from build123d import *

# Parameters (mm, degrees)
SKETCH_1_W          = 147
SKETCH_1_H          = 20
EXTRUDE_1_DEPTH     = 2
CUT_EXTRUDE_1_DEPTH = 3
SKETCH_3_R          = 1
CUT_EXTRUDE_2_DEPTH = 3
SKETCH_4_R          = 1.75
CUT_EXTRUDE_3_DEPTH = 3
CUT_EXTRUDE_4_DEPTH = 3


with BuildPart() as part:
    # 草图1 → 凸台-拉伸1 (new body)
    with BuildSketch(Plane.XY):
        Rectangle(SKETCH_1_W, SKETCH_1_H)
    extrude(amount=EXTRUDE_1_DEPTH)

    # 草图2 → 切除-拉伸1 (cut)
    with BuildSketch(Plane.XY.offset(2)):
        Polygon((30.510902349, 3.396971992), (30.740864968, 1.209023822), (45.658693398, 2.776950771), (45.428730779, 4.964898941), align=None)
    cut_extrude_1 = extrude(amount=-CUT_EXTRUDE_1_DEPTH, mode=Mode.SUBTRACT)

    # 草图3 → 切除-拉伸2 (cut, through all)
    with BuildSketch(Plane.XY.offset(2)):
        with Locations((31.505424244, 3.501500455)):
            Circle(SKETCH_3_R)
        with Locations((31.735386863, 1.313552286)):
            Circle(SKETCH_3_R)
        with Locations((44.434208884, 4.860370478)):
            Circle(SKETCH_3_R)
        with Locations((44.664171503, 2.672422308)):
            Circle(SKETCH_3_R)
    cut_extrude_2 = extrude(amount=-CUT_EXTRUDE_2_DEPTH, mode=Mode.SUBTRACT)

    # 镜向1: 切除-拉伸1, 切除-拉伸2 across plane
    add(cut_extrude_1.mirror(Plane(origin=(0, 0, 0), x_dir=(0, 0, 1), z_dir=(1, 0, 0))), mode=Mode.SUBTRACT)
    add(cut_extrude_2.mirror(Plane(origin=(0, 0, 0), x_dir=(0, 0, 1), z_dir=(1, 0, 0))), mode=Mode.SUBTRACT)

    # 草图4 → 切除-拉伸3 (cut, through all)
    with BuildSketch(Plane(origin=(0, 0, 0), x_dir=(-1, 0, 0), z_dir=(0, 0, -1))):
        with Locations((68.5, -7)):
            Circle(SKETCH_4_R)
        with Locations((48.5, -7)):
            Circle(SKETCH_4_R)
        with Locations((-48.5, -7)):
            Circle(SKETCH_4_R)
        with Locations((-68.5, -7)):
            Circle(SKETCH_4_R)
    extrude(amount=-CUT_EXTRUDE_3_DEPTH, mode=Mode.SUBTRACT)

    # 草图5 → 切除-拉伸4 (cut, through all)
    with BuildSketch(Plane.XY.offset(2)):
        with BuildLine():
            Line((52.5, 2), (67.5, 2))
            ThreePointArc((67.5, 2), (70, -0.5), (67.5, -3))
            Line((67.5, -3), (52.5, -3))
            ThreePointArc((52.5, -3), (50, -0.5), (52.5, 2))
        make_face()
    cut_extrude_4 = extrude(amount=-CUT_EXTRUDE_4_DEPTH, mode=Mode.SUBTRACT)

    # 镜向2: 切除-拉伸4 across plane
    add(cut_extrude_4.mirror(Plane(origin=(0, 0, 0), x_dir=(0, 0, 1), z_dir=(1, 0, 0))), mode=Mode.SUBTRACT)


solid = part.part
The listing builds one solid part. Answer for the finished solid, in the listing's coordinates (mm). A direction names the side the tool comes from. Coordinates: 2 decimals unless noted, no trailing zeros. Loops run counter-clockwise (first coordinate to the right, second up) from the corner with the lowest first, then second, coordinate; pieces in that order, holes last.
1) Find section C-C on y = -7. Write down the section's boundary in (x, z), then the cut area to 3 significant figures.
2) Find section A-A on z = 1.35. Give the number of separate pieces and of enclosed holes in the cut face, then the cut area to 3 significant figures.
3) A tool of negligible diameter and unlimited length cuts with its end or side. For faces 3 (the face through (70, -0.4, 1)), 4 (the face through (-1, 0, 2)), from which of +Z, -Z, +X, -X, +Y, -Y can it reach the whole face along a straight path? Write none if from no direction.
4) Find the intervals of material crossed by L1, parallel to Y at x = 48.5, z = 0.65; L2, parallel to Y at x = 68.5, z = 1; L3, parallel to X at y = 1.25, z = 0.2, in increasing order.
5) Find section B-B on x = -48.5. Write down the section's boundary in (y, z).
6) Find section D-D on x = 48. Write down the section's boundary in (y, z), then the cut area to 3 significant figures.
7) Determine the mould class of faces 1 (the face through (-1, 0, 0)), 2 (the face through (-70, -0.4, 1)) for opening direction X: pulls with the +X half, pulls with the -X half, needs draft (parallel to the pull), parting line crosses it, or undercut.
Values:
1. outline: (-73.5, 0) - (-70.25, 0) - (-70.25, 2) - (-73.5, 2) - close; (-66.75, 0) - (-50.25, 0) - (-50.25, 2) - (-66.75, 2) - close; (-46.75, 0) - (46.75, 0) - (46.75, 2) - (-46.75, 2) - close; (50.25, 0) - (66.75, 0) - (66.75, 2) - (50.25, 2) - close; (70.25, 0) - (73.5, 0) - (73.5, 2) - (70.25, 2) - close
1. area: 266 mm2
2. separate pieces: 1
2. enclosed holes: 8
2. area: 2,630 mm2
3. face 3: +Z, -Z
3. face 4: +Z, +X, -X, +Y, -Y
4. L1: y = -10 to -8.75, -5.25 to 10
4. L2: y = -10 to -8.75, -5.25 to -2.79, 1.79 to 10
4. L3: x = -73.5 to -69.29, -50.71 to -32.73, -30.74 to 30.74, 32.73 to 50.71, 69.29 to 73.5
5. outline: (-10, 0) - (-8.75, 0) - (-8.75, 2) - (-10, 2) - close; (-5.25, 0) - (10, 0) - (10, 2) - (-5.25, 2) - close
6. outline: (-10, 0) - (-8.68, 0) - (-8.68, 2) - (-10, 2) - close; (-5.32, 0) - (10, 0) - (10, 2) - (-5.32, 2) - close
6. area: 33.3 mm2
7. face 1: needs draft
7. face 2: undercut
